Study the drawing (mm; zero at the part's minimum x, y, z) and answer. Coordinates: 2 decimals unless noted, no trailing zeros. Order: outer loops, then holes, each group sorted by start corner. A loop starts at its lowest first (then second) coordinate and runs counter-clockwise, first axis right, second up. Notation, with made-up numbers: M 7.25,68.25 L 56.25,68.25 A17 cw 56.25,75.25 Z; hole C -36,61 d1. An arc over 180 degrees is marked long. Use a Markdown table: item, result. Add a question column.
1) Each of these flat-tipped pins is pushed along its axis until it touches: pin 1 Ø1.5 at (x, z) = (8.5, 13.5) entering from +Y; pin 2 Ø1.5 at (x, z) = (9.5, 7) entering from -Y; pin 3 Ø6 at (x, z) = (2.5, 4) entering from -Y. Where does it stop, or does it pass through?
2) The mould has two halves that part along Z. Classify the marked faces 1, 2 and 3: released by +Z, released by -Z, zero draft, split by the parting line, or undercut.
3) Find the intervals of material crossed by probe 1 along Z at (x, y) = (3.5, 8); probe 2 along X at (y, z) = (14.5, 12.25), in increasing order. Write a range as [from, to].
4) Find section A-A on y = 8. Write down the section's boundary in (x, z), plus the area to 3 significant figures.
5) Find section C-C on x = 10.5. Write down the section's boundary in (y, z), plus the area to 3 significant figures.
6) Find section D-D on x = 12.5. Write down the section's boundary in (y, z), plus the area to 3 significant figures.
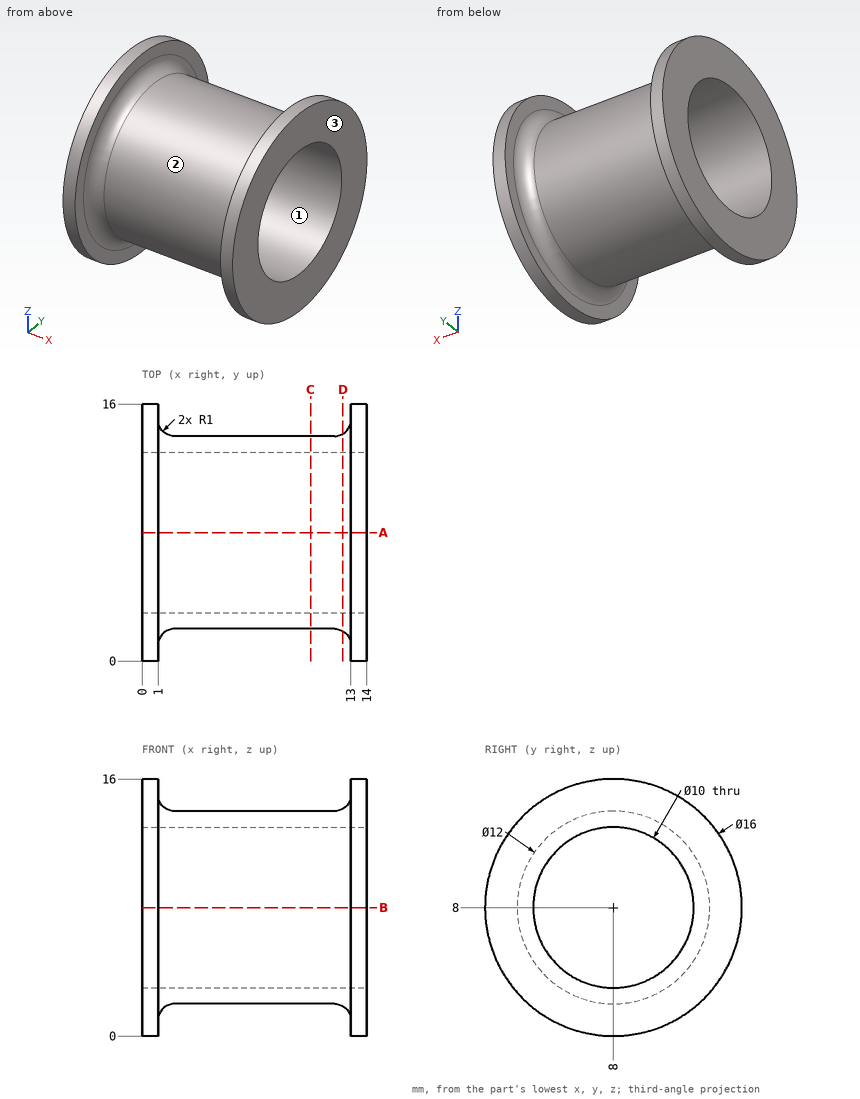
Check result:
| question | item | result |
|---|---|---|
| 1 | pin 1 | stops at y = 11.67 |
| 1 | pin 2 | stops at y = 2.01 |
| 1 | pin 3 | stops at y = 0.12 |
| 2 | face 1 | undercut |
| 2 | face 2 | split by the parting line |
| 2 | face 3 | zero draft |
| 3 | probe 1 | z = [2, 3], [13, 14] |
| 3 | probe 2 | x = [0, 1], [13, 14] |
| 4 | outline | M 0,0 L 1,0 L 1,1 A1 cw 2,2 L 12,2 A1 cw 13,1 L 13,0 L 14,0 L 14,3 L 0,3 Z; M 0,13 L 14,13 L 14,16 L 13,16 L 13,15 A1 cw 12,14 L 2,14 A1 cw 1,15 L 1,16 L 0,16 Z |
| 4 | area | 36.9 mm2 |
| 5 | outline | C 8,8 d12; hole C 8,8 d10 |
| 5 | area | 34.6 mm2 |
| 6 | outline | C 8,8 d12.27; hole C 8,8 d10 |
| 6 | area | 39.7 mm2 |
